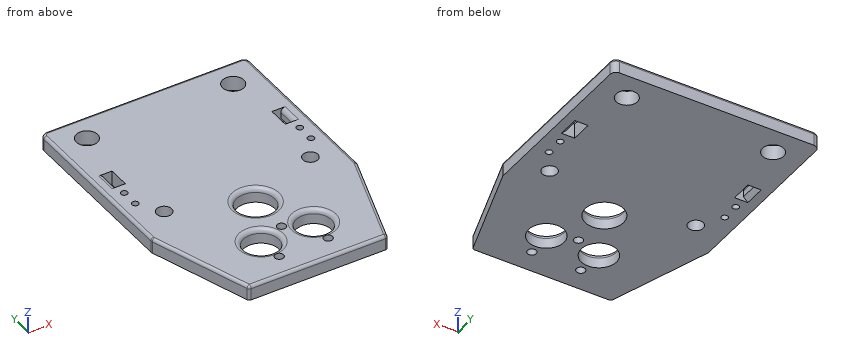
```python
from build123d import *

# Parameters (mm, degrees)
F0_R     = 1.5
F0_R_2   = 6
F0_R_3   = 2.55
F0_R_4   = 6.5
F0_R_5   = 1.125
F0_W     = 3
F0_H     = 7.25
F0_R_6   = 3.625
F1_DEPTH = 5
F2_R     = 1.5
F3_R     = 1.5
F4_SIZE  = 1.5
F5_SIZE  = 1.5
F7_R     = 1


# Not quite as in the source:
# - a fillet or chamfer that OpenCascade refuses, or shapes differently, is made with other operations: its cross-section is extruded or revolved along the edge and cut away or added


with BuildPart() as f1:
    # F0 (on Top) → F1 (new body)
    with BuildSketch(Plane.XY):
        with BuildLine():
            Line((33, 31.9801117687), (0, 31.9801117687))
            Line((0, 31.9801117687), (-33, 31.9801117687))
            ThreePointArc((-33, 31.9801117687), (-34.4142135624, 31.3943253311), (-35, 29.9801117687))
            Line((-35, 29.9801117687), (-35, 0))
            Line((-35, 0), (-35, -28.0198882313))
            ThreePointArc((-35, -28.0198882313), (-34.9746687808, -28.337194402), (-34.899316794, -28.6464628206))
            Line((-34.899316794, -28.6464628206), (-23.5597051086, -63.0198882313))
            Line((-23.5597051086, -63.0198882313), (0, -63.0198882313))
            Line((0, -63.0198882313), (23.5597051086, -63.0198882313))
            Line((23.5597051086, -63.0198882313), (34.899316794, -28.6464628206))
            ThreePointArc((34.899316794, -28.6464628206), (34.9746687808, -28.337194402), (35, -28.0198882313))
            Line((35, -28.0198882313), (35, 0))
            Line((35, 0), (35, 29.9801117687))
            ThreePointArc((35, 29.9801117687), (34.4142135624, 31.3943253311), (33, 31.9801117687))
        make_face()
        with Locations((-8.325, -55.1198882313)):
            Circle(F0_R, mode=Mode.SUBTRACT)
        with Locations((-8.95, -46.2698882313)):
            Circle(F0_R_2, mode=Mode.SUBTRACT)
        with Locations((-24.875, -19.0698882313)):
            Circle(F0_R_3, mode=Mode.SUBTRACT)
        with Locations((8.325, -55.1198882313)):
            Circle(F0_R, mode=Mode.SUBTRACT)
        with Locations((0, -43.1198882313)):
            Circle(F0_R, mode=Mode.SUBTRACT)
        with Locations((8.95, -46.2698882313)):
            Circle(F0_R_2, mode=Mode.SUBTRACT)
        with Locations((0, -29.0198882313)):
            Circle(F0_R_4, mode=Mode.SUBTRACT)
        with Locations((24.875, -19.0698882313)):
            Circle(F0_R_3, mode=Mode.SUBTRACT)
        with Locations((-29.875, -11.3948882313)):
            Circle(F0_R_5, mode=Mode.SUBTRACT)
        with Locations((-29.875, -5.3448882313)):
            Circle(F0_R_5, mode=Mode.SUBTRACT)
        with Locations((-28.7, 1.9051117687)):
            Rectangle(F0_W, F0_H, mode=Mode.SUBTRACT)
        with Locations((-24.875, 22.8551117687)):
            Circle(F0_R_6, mode=Mode.SUBTRACT)
        with Locations((29.875, -11.3948882313)):
            Circle(F0_R_5, mode=Mode.SUBTRACT)
        with Locations((29.875, -5.3448882313)):
            Circle(F0_R_5, mode=Mode.SUBTRACT)
        with Locations((28.7, 1.9051117687)):
            Rectangle(F0_W, F0_H, mode=Mode.SUBTRACT)
        with Locations((24.875, 22.8551117687)):
            Circle(F0_R_6, mode=Mode.SUBTRACT)
    extrude(amount=F1_DEPTH)

    # F2
    f2_edges = [f1.edges().sort_by_distance(p)[0] for p in [
        (30.2, 1.905112, 5),
    ]]
    fillet(f2_edges, radius=F2_R)

    # F3
    f3_edges = [f1.edges().sort_by_distance(p)[0] for p in [
        (-30.2, 1.905112, 5),
    ]]
    fillet(f3_edges, radius=F3_R)

    # F4
    f4_edges = [f1.edges().sort_by_distance(p)[0] for p in [
        (30.2, 1.905112, 0),
    ]]
    chamfer(f4_edges, length=F4_SIZE)

    # F5
    f5_edges = [f1.edges().sort_by_distance(p)[0] for p in [
        (-30.2, 1.905112, 0),
    ]]
    chamfer(f5_edges, length=F5_SIZE)

    # F6: fillet of radius 1.5 on 3 edges, made by hand

    # F6_s1 → F6_t2 (revolve, cut)
    with BuildSketch(Plane.XZ.offset(29.0198882313)):
        with BuildLine():
            ThreePointArc((6.5, 3.5), (6.9393398282, 4.5606601718), (8, 5))
            Line((8, 5), (6.5, 5))
            Line((6.5, 5), (6.5, 3.5))
        make_face()
    revolve(axis=Axis((0, -29.0198882313, 5), (0, 0, 1)), mode=Mode.SUBTRACT)

    # F6_s3 → F6_t4 (revolve, cut)
    with BuildSketch(Plane.XZ.offset(46.2698882313)):
        with BuildLine():
            ThreePointArc((-2.95, 3.5), (-2.5106601718, 4.5606601718), (-1.45, 5))
            Line((-1.45, 5), (-2.95, 5))
            Line((-2.95, 5), (-2.95, 3.5))
        make_face()
    revolve(axis=Axis((-8.95, -46.2698882313, 5), (0, 0, 1)), mode=Mode.SUBTRACT)

    # F6_s5 → F6_t6 (revolve, cut)
    with BuildSketch(Plane.XZ.offset(46.2698882313)):
        with BuildLine():
            ThreePointArc((14.95, 3.5), (15.3893398282, 4.5606601718), (16.45, 5))
            Line((16.45, 5), (14.95, 5))
            Line((14.95, 5), (14.95, 3.5))
        make_face()
    revolve(axis=Axis((8.95, -46.2698882313, 5), (0, 0, 1)), mode=Mode.SUBTRACT)

    # F7
    f7_edges = [f1.edges().sort_by_distance(p)[0] for p in [
        (29.229511, -45.833176, 5),
        (0, -63.019888, 5),
        (23.559705, -63.019888, 2.5),
        (-23.559705, -63.019888, 2.5),
        (34.974669, -28.337194, 5),
        (-34.974669, -28.337194, 5),
        (0, 31.980112, 5),
        (-34.414214, 31.394325, 5),
        (-35, 0.980112, 5),
        (-29.229511, -45.833176, 5),
        (35, 0.980112, 5),
        (34.414214, 31.394325, 5),
    ]]
    fillet(f7_edges, radius=F7_R)


solid = f1.part
```
Source: CAD feature listing. Evaluate the final solid. Frame: model axes, mm. Give positions to 0.01 mm unless a question says otherwise; leave off trailing zeros. Loops run counter-clockwise (first coordinate to the right, second up) from the corner with the lowest first, then second, coordinate; pieces in that order, holes last. Notation, with made-up numbers: (76.5, 67) -> (133.5, 67) arc R28 ccw to (133.5, 88) -> close; hole circle Ø3 at (38.25, -22.5). An arc over 180 degrees is marked (long way). Use a Markdown table: item, result. Add a question column.
(1) Section query B-B (y = 21.5). Output: boundary loops of the cut face in (x, z), then the cut area to 3 significant figures.
(2) Section query C-C (z = 2.55). Count the separate pieces of the cut face and the enclosed holes in it, then the cut area to 3 significant figures.
(3) Ray query, line 1 (Y direction, x = -8, z = 0.45); line 2 (X direction, y = -41, z = 4.1); line 3 (Y direction, x = -9.5, z = 3.15). Return the intervals inside material, ascending.
(4) First-contact query: pin 1 Ø1.5 at (x, z) = (27.5, 4.5) entering from +Y; pin 2 Ø1.5 at (x, y) = (3.5, -47.5) entering from +Z. Flat tips, straight axial feed; report the tip coordinate or a pass-through.
(5) Section query A-A (x = 0). Output: boundary loops of the cut face in (y, z), then the cut area to 3 significant figures.
Checked values:
| question | item | result |
|---|---|---|
| 1 | outline | (-35, 0) -> (-28.24, 0) -> (-28.24, 5) -> (-34, 5) arc R1 ccw to (-35, 4) -> close; (-21.51, 0) -> (21.51, 0) -> (21.51, 5) -> (-21.51, 5) -> close; (28.24, 0) -> (35, 0) -> (35, 4) arc R1 ccw to (34, 5) -> (28.24, 5) -> close |
| 1 | area | 282 mm^2 |
| 2 | separate pieces | 1 |
| 2 | enclosed holes | 16 |
| 2 | area | 5,690 mm^2 |
| 3 | line 1 | -63.02 to -56.58, -53.66 to -52.19, -40.35 to 31.98 |
| 3 | line 2 | -30.82 to -12.07, -5.83 to 5.83, 12.07 to 30.82 |
| 3 | line 3 | -63.02 to -56.05, -54.19 to -52.24, -40.3 to 31.98 |
| 4 | pin 1 | y = 31.98 |
| 4 | pin 2 | z = 4.45 |
| 5 | outline | (-63.02, 0) -> (-44.62, 0) -> (-44.62, 5) -> (-62.02, 5) arc R1 ccw to (-63.02, 4) -> close; (-41.62, 0) -> (-35.52, 0) -> (-35.52, 3.5) arc R1.5 ccw to (-37.02, 5) -> (-41.62, 5) -> close; (-22.52, 0) -> (31.98, 0) -> (31.98, 4) arc R1 ccw to (30.98, 5) -> (-21.02, 5) arc R1.5 ccw to (-22.52, 3.5) -> close |
| 5 | area | 394 mm^2 |
